Answer from the drawing. Dimensions are ordinates in mm from the lowest x, y and z of the part. A direction names the side the tool comes from. Round coordinates to 2 decimals unless told otherwise and drop trailing zeros. Write each loop counter-clockwise with the first axis right and the second up, starting at its lowest first coordinate (ties: lowest second). Pieces come first, ordered by that corner, then holes. Notation, with made-up numbers: M 37.25,-32 L 93.25,-32 A16 ccw 93.25,-21 Z; hole C 18,78.25 d7. An arc over 180 degrees is marked long. Answer as CSV lines item,"result". Start each with the question number.
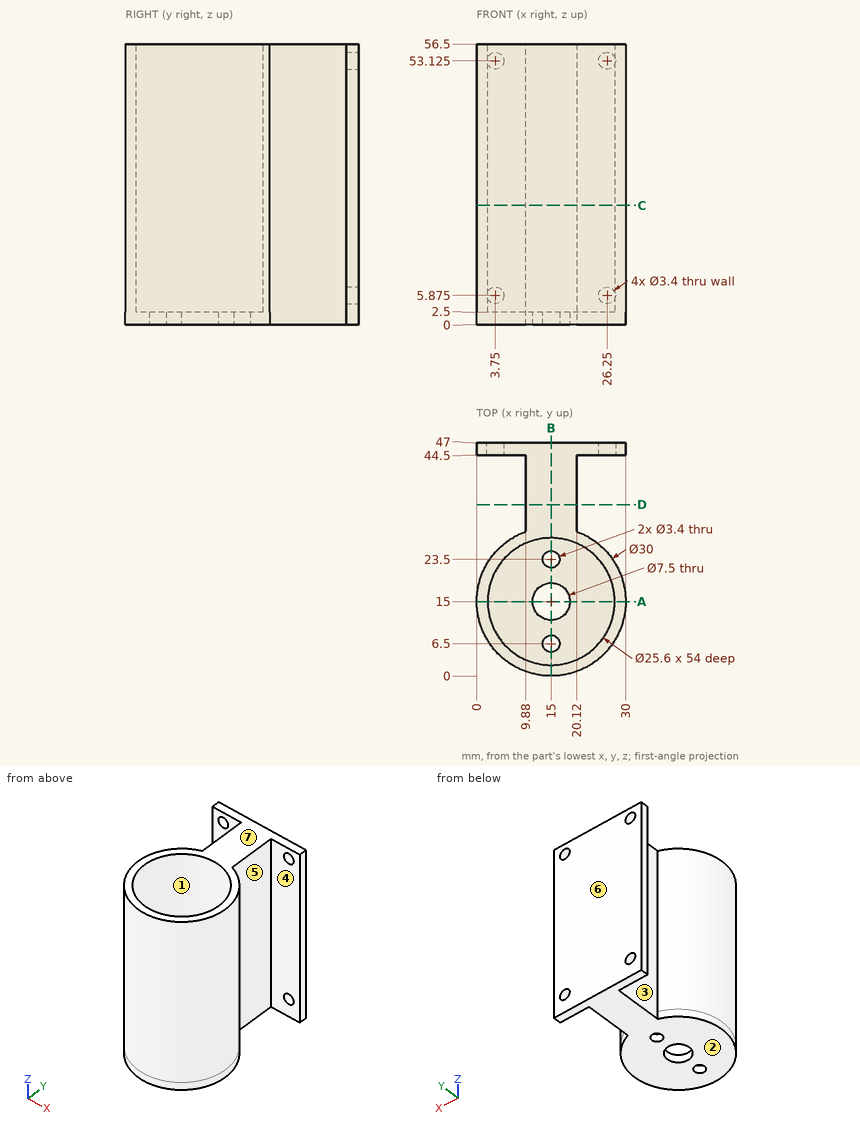
Q1. For the marked faces 1, 2, 3 and 4, determine the directions among +Z, -Z, +X, -X, +Y, -Y from which every point of the face is accessible in a straight line to the end or side of a thin tool.
Q2. Find section C-C (z = 24). Determine the outline of the cut face in (x, y), plus the area to 3 significant figures.
Q3. The mould has two halves that part along Y. Classify the marked faces 5, 6 and 7: +Y half, -Y half, draft (parallel to the pull), parting line (faces both ways), or undercut.
Q4. Find section D-D (y = 34.5). Determine the outline of the cut face in (x, z).
Q5. Find section B-B (x = 15). Determine the outline of the cut face in (y, z).
Q6. Find section A-A (y = 15). Determine the outline of the cut face in (x, z), plus the area to 3 significant figures.
Q7. Each of these flat-tipped pins is pushed along its axis until it touches: P1, Ø2, axis at x = 14, z = 44.5, coming from the -Y side; P2, Ø2, axis at x = 7, z = 17.5, coming from the -Y side; P3, Ø2, axis at x = 3.75, z = 5.875, coming from the +Y side; P4, Ø1, axis at y = 9, z = 23.5, coming from the -X side. Where does it stop, or does it pass through?
Q8. Straight lines are drawn through the part: L1, parallel to Z at x = 26.25, y = 45.15 (3 decimals); L2, parallel to Y at x = 15, z = 1; L3, parallel to Y at x = 22, z = 25. For each, find the intervals that lie inside material, in ascending order.
Reported:
1,face 1,"+Z"
1,face 2,"-Z, +X, -X, +Y, -Y"
1,face 3,"+Z, -Z, -X"
1,face 4,"+Z, -Z, +X"
2,outline,"M 0,44.5 L 9.88,44.5 L 9.88,29.1 A15 ccw long 20.12,29.1 L 20.12,44.5 L 30,44.5 L 30,47 L 0,47 Z; hole C 15,15 d25.6"
2,area,"419 mm2"
3,face 5,"undercut"
3,face 6,"+Y half"
3,face 7,"draft"
4,outline,"M 9.88,0 L 20.12,0 L 20.12,56.5 L 9.88,56.5 Z"
5,outline,"M 0,0 L 4.8,0 L 4.8,2.5 L 2.2,2.5 L 2.2,56.5 L 0,56.5 Z; M 8.2,0 L 11.25,0 L 11.25,2.5 L 8.2,2.5 Z; M 18.75,0 L 21.8,0 L 21.8,2.5 L 18.75,2.5 Z; M 25.2,0 L 47,0 L 47,56.5 L 27.8,56.5 L 27.8,2.5 L 25.2,2.5 Z"
6,outline,"M 0,0 L 11.25,0 L 11.25,2.5 L 2.2,2.5 L 2.2,56.5 L 0,56.5 Z; M 18.75,0 L 30,0 L 30,56.5 L 27.8,56.5 L 27.8,2.5 L 18.75,2.5 Z"
6,area,"294 mm2"
7,P1,"stops at y = 0"
7,P2,"stops at y = 1.73"
7,P3,"stops at y = 25.95"
7,P4,"stops at x = 1.04"
8,L1,"z = 0 to 4.175, 7.575 to 51.425, 54.825 to 56.5"
8,L2,"y = 0 to 4.8, 8.2 to 11.25, 18.75 to 21.8, 25.2 to 47"
8,L3,"y = 1.73 to 4.28, 25.72 to 28.27, 44.5 to 47"
